CAD build for the part. Positions are in the model's coordinates, mm. A direction names the side the tool comes from. Give positions to 0.01 mm unless a question says otherwise; leave off trailing zeros. Order: outer loops, then holes, each group sorted by start corner. A loop starts at its lowest first (then second) coordinate and runs counter-clockwise, first axis right, second up.
Item 1: Wall check: L1, parallel to Z at x = 98, y = 93; L2, parallel to X at y = -11.5, z = 10; L3, parallel to Y at x = 206, z = 23. Give the ranges that are in metal, low to high.
Item 2: Band-saw the part on A-A on y = 42.5. Give the cut face in (x, z), plus the area to 3 significant figures.
Item 3: Which spindle directions (+Z, -Z, +X, -X, +Y, -Y) get a long thin tool onto all of the face, cutting with end or side? Do faces 5 (the flat face through (152, -1, 25)), 6 (the flat face through (63, -24, 25.4)), 7 (the flat face through (228.73, -0.71, 18.09)). Say none if no direction does.
Item 4: Band-saw the part on C-C on x = 136. Count the separate pieces of the cut face and the enclosed holes in it, plus the area to 3 significant figures.
Item 5: Flat gauge pins, fed straight in: P1, Ø10, axis at y = -2, z = 15, coming from the -X side; P2, Ø3, axis at y = -77, z = 95, coming from the -X side; P3, Ø1, axis at y = -54.5, z = 79.5, coming from the -X side. Where does each tip first touch, or does it go through?
Item 6: Band-saw the part on B-B on y = 0. Give the cut face in (x, z), plus the area to 3 significant figures.
Item 7: Two-plate mould, pull along Y, no slides. Class faces 1 (the cylindrical face through (76.194, -0.559, 12.878)), 2 (the flat face through (155.6, -0.7, 91.2)), 3 (the flat face through (183.95, -1.42, 80.57)), 4 (the flat face through (132, 101.6, 41)): released by +Y, released by -Y, zero draft, split by the parting line, or undercut.
```python
from build123d import *

# Parameters (mm, degrees)
F1_DEPTH = 101.6
F3_DEPTH = 50.8
F5_DEPTH = 38.1


with BuildPart() as f1:
    # F0 (on Front) → F1 (new body, symmetric)
    with BuildSketch(Plane.XZ):
        Polygon((0, 25.4), (0, 0), (127, 0), (177.8, 50.8), (228.6, 0), (246.560512, 17.960512), (119.560512, 144.960512), (101.6, 127), (152.4, 76.2), (101.6, 25.4), align=None)
    extrude(amount=F1_DEPTH, both=True)

    # F2 (on face) → F3 (cut)
    with BuildSketch(Plane(origin=(132.260512, 0, 132.260512), x_dir=(0.707107, 0, -0.707107), z_dir=(0.707107, 0, 0.707107))):
        with BuildLine():
            ThreePointArc((123.54461, -76.2), (141.505122, -68.760512), (148.94461, -50.8))
            Line((148.94461, -50.8), (148.94461, 50.8))
            ThreePointArc((148.94461, 50.8), (141.505122, 68.760512), (123.54461, 76.2))
            ThreePointArc((123.54461, 76.2), (105.584098, 68.760512), (98.14461, 50.8))
            Line((98.14461, 50.8), (98.14461, -50.8))
            ThreePointArc((98.14461, -50.8), (105.584098, -68.760512), (123.54461, -76.2))
        make_face()
        with BuildLine():
            Line((-5.260512, 50.8), (-5.260512, -50.8))
            ThreePointArc((-5.260512, -50.8), (2.178976, -68.760512), (20.139488, -76.2))
            ThreePointArc((20.139488, -76.2), (38.1, -68.760512), (45.539488, -50.8))
            Line((45.539488, -50.8), (45.539488, 50.8))
            ThreePointArc((45.539488, 50.8), (38.1, 68.760512), (20.139488, 76.2))
            ThreePointArc((20.139488, 76.2), (2.178976, 68.760512), (-5.260512, 50.8))
        make_face()
    extrude(amount=-F3_DEPTH, mode=Mode.SUBTRACT)

    # F4 (on face) → F5 (cut)
    with BuildSketch(Plane.XY.offset(25.4)):
        with BuildLine():
            Line((0, -25.4), (50.8, -25.4))
            ThreePointArc((50.8, -25.4), (76.2, 0), (50.8, 25.4))
            Line((50.8, 25.4), (0, 25.4))
            Line((0, 25.4), (0, -25.4))
        make_face()
    extrude(amount=-F5_DEPTH, mode=Mode.SUBTRACT)


solid = f1.part
```
The answers:
1. L1: z = 0 to 25.4
1. L2: x = 73.45 to 137, 220.64 to 238.6
1. L3: y = -101.6 to -75.52, 75.52 to 101.6
2. outline: (0, 0) - (127, 0) - (177.8, 50.8) - (183.7, 44.9) - (201.66, 62.86) - (164.46, 100.06) - (146.5, 82.1) - (152.4, 76.2) - (101.6, 25.4) - (0, 25.4) - close; (101.6, 127) - (110.58, 118.02) - (128.54, 135.98) - (119.56, 144.96) - close; (219.62, 8.98) - (228.6, 0) - (246.56, 17.96) - (237.58, 26.94) - close
2. area: 7,470 mm2
3. face 5: -Z, +Y, -Y
3. face 6: +Z, -X, +Y, -Y
3. face 7: +Z
4. separate pieces: 3
4. enclosed holes: 0
4. area: 12,200 mm2
5. P1: stops at x = 75.22
5. P2: stops at x = 132.1
5. P3: stops at x = 148.6
6. outline: (76.2, 0) - (127, 0) - (177.8, 50.8) - (183.7, 44.9) - (201.66, 62.86) - (164.46, 100.06) - (146.5, 82.1) - (152.4, 76.2) - (101.6, 25.4) - (76.2, 25.4) - close; (101.6, 127) - (110.58, 118.02) - (128.54, 135.98) - (119.56, 144.96) - close; (219.62, 8.98) - (228.6, 0) - (246.56, 17.96) - (237.58, 26.94) - close
6. area: 5,530 mm2
7. face 1: undercut
7. face 2: undercut
7. face 3: zero draft
7. face 4: released by +Y
